from build123d import *

# Parameters (mm, degrees)
SKETCH1_R           = 125
SKETCH1_R_2         = 16
SKETCH1_R_3         = 1.5
SKETCH1_W           = 20
SKETCH1_H           = 65.2
BOSS_EXTRUDE1_DEPTH = 5


with BuildPart() as part:
    # Sketch1 → Boss-Extrude1 (new body)
    with BuildSketch(Plane(origin=(0, 0, 0), x_dir=(1, 0, 0), z_dir=(0, 1, 0))):
        with Locations((0, -6.988561475)):
            Circle(SKETCH1_R)
        with Locations((0, -86.988561475)):
            Circle(SKETCH1_R_2, mode=Mode.SUBTRACT)
        with Locations((60, 18.011438525)):
            Circle(SKETCH1_R_3, mode=Mode.SUBTRACT)
        with Locations((60, 67.011438525)):
            Circle(SKETCH1_R_3, mode=Mode.SUBTRACT)
        with Locations((29, 67.011438525)):
            Circle(SKETCH1_R_3, mode=Mode.SUBTRACT)
        with Locations((29, 18.011438525)):
            Circle(SKETCH1_R_3, mode=Mode.SUBTRACT)
        with Locations((-60, 18.011438525)):
            Circle(SKETCH1_R_3, mode=Mode.SUBTRACT)
        with Locations((-29, 18.011438525)):
            Circle(SKETCH1_R_3, mode=Mode.SUBTRACT)
        with Locations((-29, 67.011438525)):
            Circle(SKETCH1_R_3, mode=Mode.SUBTRACT)
        with Locations((-60, 67.011438525)):
            Circle(SKETCH1_R_3, mode=Mode.SUBTRACT)
        with Locations((79.5, 35.555700821)):
            Rectangle(SKETCH1_W, SKETCH1_H, mode=Mode.SUBTRACT)
        with Locations((-79.5, 35.555700821)):
            Rectangle(SKETCH1_W, SKETCH1_H, mode=Mode.SUBTRACT)
    extrude(amount=BOSS_EXTRUDE1_DEPTH)


solid = part.part
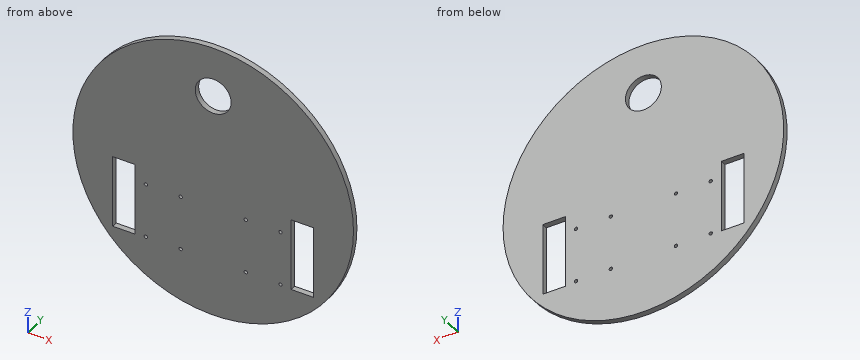
Part model, mm, in its own coordinate system. Coordinates: 2 decimals unless noted, no trailing zeros. Order: outer loops, then holes, each group sorted by start corner. A loop starts at its lowest first (then second) coordinate and runs counter-clockwise, first axis right, second up.
(1) Slice it at C-C, the plane y = 4.1. State how many separate pieces and enclosed holes the cut face has, and give its area (3 significant figures).
Check sheet entries:
separate pieces: 1
enclosed holes: 11
area: 45,600 mm2
(2) Pin check, flat tips, straight feed: pin 1 Ø1.5 at (y, z) = (3, -28) entering from -X; pin 2 Ø1 at (y, z) = (1, -44.5) entering from -X; pin 3 Ø1.5 at (x, y) = (-76, 2.5) entering from -Z; pin 4 Ø2.5 at (x, z) = (-29, -67.01) entering from -Y. Stop position of each tip, or through.
Check sheet entries:
pin 1: stops at x = -120.22
pin 2: stops at x = -114.13
pin 3: stops at z = -92.82
pin 4: passes through
(3) Slice it at A-A, the plane x = 0. Write the cut outline in (y, z), and give its area (3 significant figures).
Check sheet entries:
outline: (0, -118.01) - (5, -118.01) - (5, 70.99) - (0, 70.99) - close; (0, 102.99) - (5, 102.99) - (5, 131.99) - (0, 131.99) - close
area: 1,090 mm2
(4) Slice it at D-D, the plane z = 37. Write the cut outline in (x, y), and give its area (3 significant figures).
Check sheet entries:
outline: (-121.34, 0) - (121.34, 0) - (121.34, 5) - (-121.34, 5) - close
area: 1,210 mm2
(5) Probe L1, parallel to Z at x = 29, y = 1.95; L2, parallel to X at y = 3.65, z = -57.5; L3, parallel to Z at x = -60, y = 1.2. List the from-to ranges inside material, lowest first.
Check sheet entries:
L1: z = -114.6 to -68.51, -65.51 to -19.51, -16.51 to 128.58
L2: x = -107.08 to -89.5, -69.5 to 69.5, 89.5 to 107.08
L3: z = -102.67 to -68.51, -65.51 to -19.51, -16.51 to 116.65
(6) Slice it at B-B, the plane z = -31.5. Write the cut outline in (x, y), and give its area (3 significant figures).
Check sheet entries:
outline: (-118.93, 0) - (-89.5, 0) - (-89.5, 5) - (-118.93, 5) - close; (-69.5, 0) - (69.5, 0) - (69.5, 5) - (-69.5, 5) - close; (89.5, 0) - (118.93, 0) - (118.93, 5) - (89.5, 5) - close
area: 989 mm2
